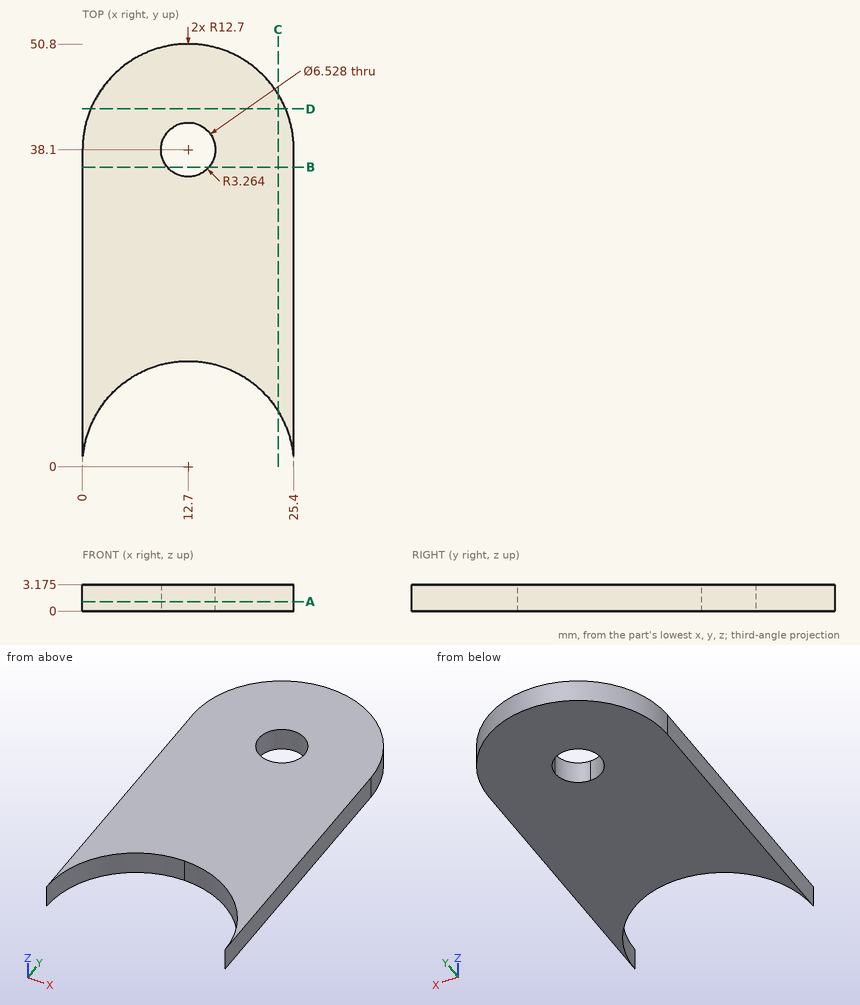
For this review, use the dimensioned drawing (mm, ordinates from the lowest corner) and the shaded views. Give positions to 0.01 mm unless a question says otherwise; leave off trailing zeros. Order: outer loops, then holes, each group sorted by start corner. A loop starts at its lowest first (then second) coordinate and runs counter-clockwise, first axis right, second up.
1) Take a section at B-B (y = 36). Give the boundary of the cut face in (x, z) (1 decimal).
2) Take a section at A-A (z = 1.15). Give the boundary of the cut face in (x, y), then the cut area to 3 significant figures.
3) Take a section at C-C (x = 23.5). Give the boundary of the cut face in (y, z) (3 decimals), then the cut area to 3 significant figures.
4) Wall thickness on line 1 (X direction, y = 38.1, z = 1.45); line 2 (X direction, y = 8.5, z = 1.4) (1 decimal); line 3 (Y direction, x = 14.25, z = 3) (1 decimal): over which ranges is each line inside the solid? List them lowest first.
5) Take a section at D-D (y = 43). Give the boundary of the cut face in (x, z) (1 decimal), then the cut area to 3 significant figures.
Derived:
1. outline: (0, 0) - (10.2, 0) - (10.2, 3.2) - (0, 3.2) - close; (15.2, 0) - (25.4, 0) - (25.4, 3.2) - (15.2, 3.2) - close
2. outline: (0, 0) arc R12.7 cw to (25.4, 0) - (25.4, 38.1) arc R12.7 ccw to (0, 38.1) - close; hole circle Ø6.53 at (12.7, 38.1)
2. area: 934 mm2
3. outline: (6.682, 0) - (44.782, 0) - (44.782, 3.175) - (6.682, 3.175) - close
3. area: 121 mm2
4. line 1: x = 0 to 9.44, 15.96 to 25.4
4. line 2: x = 0 to 3.3, 22.1 to 25.4
4. line 3: y = 12.6 to 35.2, 41 to 50.7
5. outline: (1, 0) - (24.4, 0) - (24.4, 3.2) - (1, 3.2) - close
5. area: 74.4 mm2
